Work out the finished part from the listing and answer in its coordinate system (mm). Face numbers are marked on the shaded views. A direction names the side the tool comes from. Round coordinates to 2 decimals unless told otherwise and drop trailing zeros. Order: outer loops, then holes, each group sorted by start corner. A loop starts at its lowest first (then second) coordinate and runs counter-clockwise, first axis right, second up. Notation, with made-up numbers: (4.25, 26.5) - (37.25, 26.5) arc R23 ccw to (37.25, 41.5) - close; hole circle Ø2 at (3.5, 11). An arc over 180 degrees is marked (long way). Put each result on its own line as item: value.
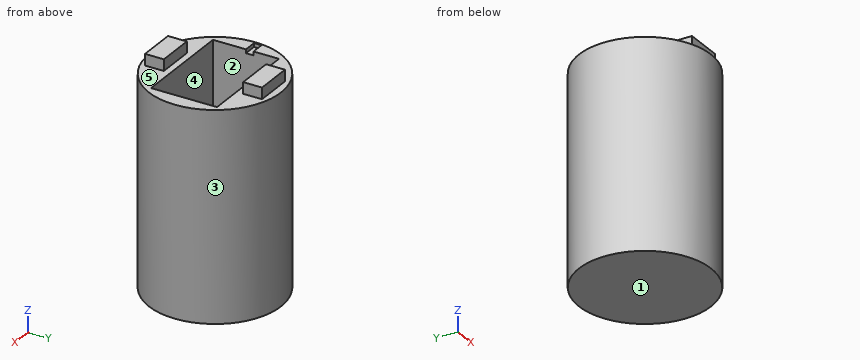
```python
from build123d import *

# Parameters (mm, degrees)
BOX003_W       = 4
BOX003_H       = 2
BOX003_DEPTH   = 2
BOX_W          = 27
BOX_H          = 17.5
BOX_DEPTH      = 53
CYLINDER_R     = 17.5
CYLINDER_DEPTH = 55
BOX001_W       = 10
BOX001_H       = 5
BOX001_DEPTH   = 3
BOX002_W       = 10
BOX002_H       = 5
BOX002_DEPTH   = 3


with BuildPart() as box003:
    # Box003 → Box003 (new body)
    with BuildSketch(Plane(origin=(-17, 0, 54), x_dir=(1, 0, 0), z_dir=(0, 0, 1))):
        with Locations((2, 1)):
            Rectangle(BOX003_W, BOX003_H)
    extrude(amount=BOX003_DEPTH)


with BuildPart() as box:
    # Box → Box (new body)
    with BuildSketch(Plane(origin=(-13.5, -8.75, 2), x_dir=(1, 0, 0), z_dir=(0, 0, 1))):
        with Locations((13.5, 8.75)):
            Rectangle(BOX_W, BOX_H)
    extrude(amount=BOX_DEPTH)


with BuildPart() as cut:
    # Cylinder → Cylinder (new body)
    with BuildSketch(Plane.XY):
        Circle(CYLINDER_R)
    extrude(amount=CYLINDER_DEPTH)

    # Cut: cut Box
    add(box.part, mode=Mode.SUBTRACT)


with BuildPart() as fusion:
    # Box001 → Box001 (new body)
    with BuildSketch(Plane(origin=(-5, 10.5, 55), x_dir=(1, 0, 0), z_dir=(0, 0, 1))):
        with Locations((5, 2.5)):
            Rectangle(BOX001_W, BOX001_H)
    extrude(amount=BOX001_DEPTH)

    # Fusion: union Cut
    add(cut.part)


with BuildPart() as cut001:
    # Box002 → Box002 (new body)
    with BuildSketch(Plane(origin=(-5, -15.5, 55), x_dir=(1, 0, 0), z_dir=(0, 0, 1))):
        with Locations((5, 2.5)):
            Rectangle(BOX002_W, BOX002_H)
    extrude(amount=BOX002_DEPTH)

    # Fusion001: union Fusion
    add(fusion.part)

    # Cut001: cut Box003
    add(box003.part, mode=Mode.SUBTRACT)


solid = cut001.part
```
1) Straight lines are drawn through the part: L1, parallel to Y at x = 0.5, z = 26; L2, parallel to X at y = 14, z = 17; L3, parallel to Z at x = -7, y = -15. For each, find the intervals that lie inside material, in ascending order. Write a range as from..to.
Findings below:
L1: y = -17.49..-8.75, 8.75..17.49
L2: x = -10.5..10.5
L3: z = 0..55
2) Given pin 1 Ø3.5 at (y, z) = (13.5, 56.5) entering from +X; pin 2 Ø2.5 at (y, z) = (-14, 56) entering from -X; pin 3 Ø1.5 at (x, z) = (-1.5, 56) entering from -Y, each flat-ended and moving along its own axis, determine where each tip first touches the part or whether it passes through.
Findings below:
pin 1: stops at x = 12.15
pin 2: stops at x = -11.43
pin 3: stops at y = -15.5
3) A cutting plane is placed at B-B on z = 45. Write down the section's boundary in (x, y).
Findings below:
outline: circle Ø35 at (0, 0); hole (-13.5, -8.75) - (13.5, -8.75) - (13.5, 8.75) - (-13.5, 8.75) - close
4) A cutting plane is placed at A-A on x = 0. Write down the section's boundary in (y, z).
Findings below:
outline: (-17.5, 0) - (17.5, 0) - (17.5, 55) - (15.5, 55) - (15.5, 58) - (10.5, 58) - (10.5, 55) - (8.75, 55) - (8.75, 2) - (-8.75, 2) - (-8.75, 55) - (-10.5, 55) - (-10.5, 58) - (-15.5, 58) - (-15.5, 55) - (-17.5, 55) - close
5) For a pull along X with two mould halves and no side action, classify the marked faces 3, 4 and 5 as pulls with the +X half, pulls with the -X half, needs draft (parallel to the pull), parting line crosses it, or undercut.
Findings below:
face 3: parting line crosses it
face 4: undercut
face 5: needs draft
6) A cutting plane is placed at D-D on x = -10.5. Write down the section's boundary in (y, z), then the cut area to 4 significant figures.
Findings below:
outline: (-14, 0) - (14, 0) - (14, 55) - (8.75, 55) - (8.75, 2) - (-8.75, 2) - (-8.75, 55) - (-14, 55) - close
area: 612.5 mm2
7) A cutting plane is placed at C-C on y = 1. Write down the section's boundary in (x, z), then the cut area to 3 significant figures.
Findings below:
outline: (-17.47, 0) - (17.47, 0) - (17.47, 55) - (13.5, 55) - (13.5, 2) - (-13.5, 2) - (-13.5, 54) - (-17, 54) - (-17, 55) - (-17.47, 55) - close
area: 487 mm2
8) For the marked faces 1 and 2, determine the directions among +Z, -Z, +X, -X, +Y, -Y from which every point of the face is accessible in a straight line to the end or side of a thin tool.
Findings below:
face 1: -Z, +X, -X, +Y, -Y
face 2: +Z
